Autodesk Inventor part; units mm, degrees
ref_plane "YZ Plane" through (0, 0, 0) normal (1, 0, 0) x (0, 1, 0)
ref_plane "XZ Plane" through (0, 0, 0) normal (0, 1, 0) x (-1, 0, 0)
ref_plane "XY Plane" through (0, 0, 0) normal (0, 0, 1) x (1, 0, 0)
sketch "Sketch1" plane through (0, 0, 0) normal (0, 0, 1) x (1, 0, 0)
  line L0 (0, 0) -> (-31.75, 0)
  line L1 (-31.75, 0) -> (-31.75, 155.575)
  line L2 (-31.75, 155.575) -> (0, 155.575)
  line L3 (0, 155.575) -> (0, 0)
  circle A0 centre (-53.975, 55.5625) radius 9.525 construction
  line L4 (-62.4238, 59.9607) -> (-12.6501, 155.575)
  point P0 (-31.75, 118.8844)
  dimension "d2" = 19.05
  dimension "d0" = 31.75
  dimension "d1" = 155.575
  dimension "d3" = 53.975
  dimension "d4" = 55.5625
  dimension "d5" = 27.5
extrude "Extrusion1" add sketch "Sketch1" along normal blind 6.35 contours L0 L1 L4 L2 L3
properties part number "Side Plate" material "UHMW, White"
Geometry check sheet. Reference: the model listing, model coordinates, mm. Round coordinates to 2 decimals unless told otherwise and drop trailing zeros. Write each loop counter-clockwise with the first axis right and the second up, starting at its lowest first coordinate (ties: lowest second). Pieces come first, ordered by that corner, then holes. Notation, with made-up numbers: (4, 81.5) - (61, 81.5) arc R13 ccw to (61, 100.5) - close; hole circle Ø10 at (28, -26.75). An arc over 180 degrees is marked (long way). Write each question's results on one line, items separated by ' | '.
(1) Sectioned sample at B-B, the plane x = -14. Enter the section's corners in (y, z).
Computed:
outline: (0, 0) - (152.98, 0) - (152.98, 6.35) - (0, 6.35) - close
(2) Sectioned sample at C-C, the plane y = 141. Enter the section's corners in (x, z), plus the area to 3 significant figures.
Computed:
outline: (-20.24, 0) - (0, 0) - (0, 6.35) - (-20.24, 6.35) - close | area: 129 mm^2
(3) Sectioned sample at A-A, the plane z = 1.25. Enter the section's corners in (x, y) (3 decimals).
Computed:
outline: (-31.75, 0) - (0, 0) - (0, 155.575) - (-12.65, 155.575) - (-31.75, 118.884) - close
(4) Thickness scan on probe 1 along Y at (x, z) = (-22, 6.25); probe 2 along X at (y, z) = (143, 0.5); probe 3 along Y at (x, z) = (-20, 5.25). Record the ranges inside material, lowest first. Write a range as from..to.
Computed:
probe 1: y = 0..137.61 | probe 2: x = -19.2..0 | probe 3: y = 0..141.46
(5) Depth check by flat-ended pin: pin 1 Ø1.5 at (x, z) = (-27.5, 5.5) entering from +Y. Enter the tip coordinate at first touch or a pass-through.
Computed:
pin 1: stops at y = 128.49
